For this review, take the finished solid that the model builds, in its own axes (mm). Coordinates: 2 decimals unless noted, no trailing zeros. Loops run counter-clockwise (first coordinate to the right, second up) from the corner with the lowest first, then second, coordinate; pieces in that order, holes last. Notation, with made-up numbers: (69.25, -23.75) -> (127.25, -23.75) arc R13 cw to (127.25, -1.75) -> close; hole circle Ø7 at (85, -17.75). An arc over 180 degrees is marked (long way). Use a Markdown table: item, result.
Autodesk Inventor part; units mm, degrees
ref_plane "Work Plane1" through (0, 12, 0) normal (0, 1, 0) x (1, 0, 0)
ref_plane "YZ Plane" through (0, 0, 0) normal (1, 0, 0) x (0, 1, 0)
ref_plane "XZ Plane" through (0, 0, 0) normal (0, 1, 0) x (-1, 0, 0)
sketch "Sketch1" plane through (0, 0, 0) normal (0, 1, 0) x (-1, 0, 0)
  line L0 (60, -40) -> (-60, -40)
  line L1 (-65, -35) -> (-65, 35)
  line L2 (-60, 40) -> (60, 40)
  line L3 (65, 35) -> (65, -35)
  arc A0 (60, -40) -> (65, -35) centre (60, -35) ccw
  arc A1 (-65, -35) -> (-60, -40) centre (-60, -35) ccw
  arc A2 (-60, 40) -> (-65, 35) centre (-60, 35) ccw
  arc A3 (65, 35) -> (60, 40) centre (60, 35) ccw
  line L4 (60, -37.5) -> (-60, -37.5)
  line L5 (-62.5, -35) -> (-62.5, 35)
  line L6 (-60, 37.5) -> (60, 37.5)
  line L7 (62.5, 35) -> (62.5, -35)
  arc A4 (62.5, 35) -> (60, 37.5) centre (60, 35) ccw
  arc A5 (60, -37.5) -> (62.5, -35) centre (60, -35) ccw
  arc A6 (-62.5, -35) -> (-60, -37.5) centre (-60, -35) ccw
  arc A7 (-60, 37.5) -> (-62.5, 35) centre (-60, 35) ccw
  point P0 (0, 0)
  point P1 (-65, 40)
  point P2 (-65, -40)
  point P3 (65, 40)
  dimension "d0" = 130
  dimension "d1" = 80
  dimension "d2" = 5
  dimension "d3" = 2.5
  dimension "d4" = 2.5
  dimension "d5" = 2.5
  dimension "d6" = 2.5
  dimension "d7" = 2.5
  dimension "d32" = 65
  dimension "d33" = 40
extrude "Extrusion1" add sketch "Sketch1" along normal blind 24
sketch "Sketch2" plane through (0, 24, 0) normal (0, 1, 0) x (1, 0, 0)
  line L0 (-60, -38.5) -> (60, -38.5)
  line L1 (63.5, -35) -> (63.5, 35)
  line L2 (60, 38.5) -> (-60, 38.5)
  line L3 (-63.5, 35) -> (-63.5, -35)
  line L4 (-60, 37.5) -> (60, 37.5)
  line L5 (62.5, 35) -> (62.5, -35)
  line L6 (60, -37.5) -> (-60, -37.5)
  line L7 (-62.5, -35) -> (-62.5, 35)
  arc A0 (-63.5, -35) -> (-60, -38.5) centre (-60, -35) ccw
  arc A1 (-60, 38.5) -> (-63.5, 35) centre (-60, 35) ccw
  arc A2 (63.5, 35) -> (60, 38.5) centre (60, 35) ccw
  arc A3 (60, -38.5) -> (63.5, -35) centre (60, -35) ccw
  point P0 (0, 0)
  dimension "d10" = 1
  dimension "d11" = 1
  dimension "d12" = 1
  dimension "d13" = 1
  dimension "d14" = 3.5
extrude "Extrusion2" cut sketch "Sketch2" against normal blind 1
ref_plane "Work Plane1" through (0, 12, 0) normal (0, 1, 0) x (1, 0, 0)
mirror "Mirror1" about plane through (0, 12, 0) normal (0, 1, 0) of "Extrusion2"
sketch "Sketch3" plane through (0, 23, 0) normal (0, 1, 0) x (1, 0, 0)
  line L0 (-56.5, 37.5) -> (-62.5, 37.5)
  line L1 (-62.5, 37.5) -> (-62.5, 31.5)
  line L2 (-62.5, 31.5) -> (-56.5, 31.5)
  line L3 (-56.5, 31.5) -> (-56.5, 37.5)
  line L4 (60, 37.5) -> (-60, 37.5)
  line L5 (-62.5, 35) -> (-62.5, -35)
  circle A0 centre (-60, 35) radius 2.4
  arc A1 (-60, 37.5) -> (-62.5, 35) centre (-60, 35) ccw
  point P0 (0, 0)
  dimension "d18" = 6
  dimension "d19" = 6
  dimension "d20" = 4.8
extrude "Extrusion3" add sketch "Sketch3" against normal up to surface (22 mm away)
fillet "Fillet2" radius 3.5 1 edges at (-56.5, 12, -31.5)
mirror "Mirror2" about plane through (0, 0, 0) normal (0, 0, 1) of "Extrusion3", "Fillet2"
mirror "Mirror3" about plane through (0, 0, 0) normal (1, 0, 0) of "Fillet2", "Extrusion3", "Mirror2"
sketch "Sketch7" plane through (60, 0, -40) normal (0, 0, -1) x (-1, 0, 0)
  line L0 (13, 22.6) -> (75, 22.6)
  line L1 (75, 22.6) -> (75, 7.6)
  line L2 (75, 7.6) -> (13, 7.6)
  line L3 (13, 7.6) -> (13, 22.6)
  line L4 (-5, 0) -> (-5, 24)
  line L5 (0, 0) -> (120, 0)
  point P0 (60, 0)
  dimension "d35" = 62
  dimension "d36" = 15
  dimension "d37" = 18
  dimension "d38" = 7.6
extrude "Extrusion4" cut sketch "Sketch7" against normal blind 24
sketch "Sketch8" plane through (-56.5, 1, -37.5) normal (0, 0, 1) x (1, 0, 0)
  line L0 (-3.5, 22) -> (116.5, 22)
  line L1 (3.6019, 22) -> (106.4534, 22)
  line L2 (106.4534, 22) -> (106.4534, 1)
  line L3 (106.4534, 1) -> (3.6019, 1)
  line L4 (3.6019, 1) -> (3.6019, 22)
  point P0 (56.5, -1)
  dimension "d43" = 21
extrude "Extrusion5" cut sketch "Sketch8" against normal blind 1
sketch "Sketch9" plane through (60, 0, -40) normal (0, 0, -1) x (-1, 0, 0)
  line L0 (83, 14) -> (92.2, 14)
  line L1 (92.2, 14) -> (92.2, 2.6)
  line L2 (92.2, 2.6) -> (83, 2.6)
  line L3 (83, 2.6) -> (83, 14)
  line L4 (75, 22.6) -> (75, 7.6)
  line L5 (100.2, 4.5) -> (110.2, 4.5)
  line L6 (110.2, 4.5) -> (110.2, 19.5)
  line L7 (110.2, 19.5) -> (100.2, 19.5)
  line L8 (100.2, 19.5) -> (100.2, 4.5)
  circle A0 centre (87.6, 19) radius 1.5
  line L9 (10.0466, 2) -> (112.8981, 2)
  line L10 (0, 24) -> (120, 24)
  point P0 (60, 0)
  point P1 (83, 8.3)
  dimension "d44" = 8
  dimension "d45" = 9.2
  dimension "d46" = 11.4
  dimension "d47" = 10
  dimension "d48" = 15
  dimension "d49" = 8
  dimension "d50" = 3
  dimension "d51" = 5
  dimension "d54" = 0.6
  dimension "d55" = 4.5
extrude "Extrusion6" cut sketch "Sketch9" against normal blind 2
sketch "Sketch10" plane through (0, 24, 0) normal (0, 1, 0) x (1, 0, 0)
  line L0 (-65.5813, 44.518) -> (-55.4636, 44.518)
  line L1 (-55.4636, 44.518) -> (-55.4636, 27.5938)
  line L2 (-55.4636, 27.5938) -> (54.5438, 27.5938)
  line L3 (54.5438, 27.5938) -> (54.5438, 46.5416)
  line L4 (54.5438, 46.5416) -> (69.4444, 46.5416)
  line L5 (69.4444, 46.5416) -> (73.6755, -45.2538)
  line L6 (73.6755, -45.2538) -> (-73.3076, -45.2538)
  line L7 (-73.3076, -45.2538) -> (-65.5813, 44.518)
  point P0 (0, 0)
extrude "Extrusion7" cut sketch "Sketch10" against normal through all
equation "\"d4\" = d3"
equation "\"d5\" = d3"
equation "\"d6\" = d3"
equation "\"d11\" = d10"
equation "\"d12\" = d10"
equation "\"d13\" = d10"
properties part number "front_panel"
(1) For pin 1 Ø0.8 at (x, z) = (23.5, -38) entering from +Y; pin 2 Ø4 at (x, y) = (14, 19) entering from -Z; pin 3 Ø0.5 at (x, y) = (19, 0.5) entering from +Z, all flat-tipped, find the tip position at first contact; note any pin that passes through.
Found:
| item | result |
|---|---|
| pin 1 | stops at y = 2 |
| pin 2 | passes through |
| pin 3 | stops at z = -38.5 |
(2) Take a section at D-D on x = -27.6. Write out the cut boundary in (y, z).
Found:
| item | result |
|---|---|
| outline | (0, -40) -> (2.6, -40) -> (2.6, -38.5) -> (2, -38.5) -> (2, -37.5) -> (1, -37.5) -> (1, -38.5) -> (0, -38.5) -> close; (14, -40) -> (17.5, -40) -> (17.5, -38.5) -> (14, -38.5) -> close; (20.5, -40) -> (24, -40) -> (24, -38.5) -> (20.5, -38.5) -> close |
(3) Take a section at C-C on z = -39.2. Write out the cut boundary in (x, y), plus the area to 3 significant figures.
Found:
| item | result |
|---|---|
| outline | (-55.46, 0) -> (54.54, 0) -> (54.54, 24) -> (-55.46, 24) -> close; hole (-50.2, 4.5) -> (-40.2, 4.5) -> (-40.2, 19.5) -> (-50.2, 19.5) -> close; hole (-32.2, 2.6) -> (-23, 2.6) -> (-23, 14) -> (-32.2, 14) -> close; hole circle Ø3 at (-27.6, 19); hole (-15, 7.6) -> (47, 7.6) -> (47, 22.6) -> (-15, 22.6) -> close |
| area | 1,450 mm^2 |
(4) Take a section at A-A on y = 8.75. Write out the cut boundary in (x, z), plus the area to 3 significant figures.
Found:
| item | result |
|---|---|
| outline | (-55.46, -40) -> (-50.2, -40) -> (-50.2, -38.5) -> (-52.9, -38.5) -> (-52.9, -37.5) -> (-55.46, -37.5) -> close; (-40.2, -40) -> (-32.2, -40) -> (-32.2, -38.5) -> (-40.2, -38.5) -> close; (-23, -40) -> (-15, -40) -> (-15, -38.5) -> (-23, -38.5) -> close; (47, -40) -> (54.54, -40) -> (54.54, -37.5) -> (49.95, -37.5) -> (49.95, -38.5) -> (47, -38.5) -> close |
| area | 50.4 mm^2 |
(5) For line 1 along X through (y, z) = (6.5, -39.15); line 2 along Y through (x, z) = (-27.6, -39.45); line 3 along X through (y, z) = (7.75, -39.6), list the stretches that pass through material, from the lowest coordinate up.
Found:
| item | result |
|---|---|
| line 1 | x = -55.46 to -50.2, -40.2 to -32.2, -23 to 54.54 |
| line 2 | y = 0 to 2.6, 14 to 17.5, 20.5 to 24 |
| line 3 | x = -55.46 to -50.2, -40.2 to -32.2, -23 to -15, 47 to 54.54 |
(6) Mouldability with a two-part tool opening along X and no side actions: class faces 1 (the face through (-1, 6, -40)), 2 (the face through (0, 6, -38.5)), 3 (the face through (-55.464, 12, -39)) as pulls with the +X half, pulls with the -X half, needs draft (parallel to the pull), parting line crosses it, or undercut.
Found:
| item | result |
|---|---|
| face 1 | needs draft |
| face 2 | undercut |
| face 3 | pulls with the -X half |
(7) Take a section at B-B on x = -13.5. Write out the cut boundary in (y, z), plus the area to 3 significant figures.
Found:
| item | result |
|---|---|
| outline | (0, -40) -> (7.6, -40) -> (7.6, -38.5) -> (2, -38.5) -> (2, -37.5) -> (1, -37.5) -> (1, -38.5) -> (0, -38.5) -> close; (22.6, -40) -> (24, -40) -> (24, -38.5) -> (22.6, -38.5) -> close |
| area | 14.5 mm^2 |
